from build123d import *

# Parameters (mm, degrees)
F2_DEPTH = 70


# Not quite as in the source:
# - ends of sketch curves that miss each other by under 0.0002 mm in the source are joined


with BuildPart() as f2:
    # F1 (on Front) → F2 (new body, symmetric)
    with BuildSketch(Plane.XZ):
        with BuildLine():
            Line((8.249944, 9.6642), (4.58573, 5.999986))
            Line((4.58573, 5.999986), (0.653534, 5.999986))
            ThreePointArc((0.653534, 5.999986), (0.5241245494, 5.9829489324), (0.4035341291, 5.9329987764))
            Line((0.4035341291, 5.9329987764), (-5.6e-05, 5.699986))
            Line((-5.6e-05, 5.699986), (-0.403646, 5.932999))
            ThreePointArc((-0.403646, 5.932999), (-0.653646, 5.999986), (-0.9036458709, 5.9329987764))
            Line((-0.9036458709, 5.9329987764), (-1.218942, 5.750963))
            Line((-1.218942, 5.750963), (-2.500056, 5.999986))
            Line((-2.500056, 5.999986), (-4.585842, 5.999986))
            Line((-4.585842, 5.999986), (-8.250056, 9.6642))
            Line((-8.250056, 9.6642), (-8.250056, 12.999986))
            Line((-8.250056, 12.999986), (-4.300056, 12.999986))
            ThreePointArc((-4.300056, 12.999986), (-4.0879239656, 13.0878539656), (-4.000056, 13.299986))
            Line((-4.000056, 13.299986), (-4.000056, 14.699986))
            ThreePointArc((-4.000056, 14.699986), (-4.0879239656, 14.9121180344), (-4.300056, 14.999986))
            Line((-4.300056, 14.999986), (-13.000056, 14.999986))
            ThreePointArc((-13.000056, 14.999986), (-14.4142695624, 14.4141995624), (-15.000056, 12.999986))
            Line((-15.000056, 12.999986), (-15.000056, 4.299986))
            ThreePointArc((-15.000056, 4.299986), (-14.9121880344, 4.0878539656), (-14.700056, 3.999986))
            Line((-14.700056, 3.999986), (-13.300056, 3.999986))
            ThreePointArc((-13.300056, 3.999986), (-13.0879239656, 4.0878539656), (-13.000056, 4.299986))
            Line((-13.000056, 4.299986), (-13.000056, 8.249986))
            Line((-13.000056, 8.249986), (-9.66427, 8.249986))
            Line((-9.66427, 8.249986), (-6.000056, 4.585772))
            Line((-6.000056, 4.585772), (-6.000056, 0.653576))
            ThreePointArc((-6.000056, 0.653576), (-5.9830189324, 0.5241665494), (-5.9330687764, 0.4035761291))
            Line((-5.9330687764, 0.4035761291), (-5.700056, -1.4e-05))
            Line((-5.700056, -1.4e-05), (-5.933069, -0.403604))
            ThreePointArc((-5.933069, -0.403604), (-6.000056, -0.653604), (-5.9330687764, -0.9036038709))
            Line((-5.9330687764, -0.9036038709), (-5.751033, -1.2189))
            Line((-5.751033, -1.2189), (-6.000056, -2.500014))
            Line((-6.000056, -2.500014), (-6.000056, -4.5858))
            Line((-6.000056, -4.5858), (-9.66427, -8.250014))
            Line((-9.66427, -8.250014), (-13.000056, -8.250014))
            Line((-13.000056, -8.250014), (-13.000056, -4.300014))
            ThreePointArc((-13.000056, -4.300014), (-13.0879239656, -4.0878819656), (-13.300056, -4.000014))
            Line((-13.300056, -4.000014), (-14.700056, -4.000014))
            ThreePointArc((-14.700056, -4.000014), (-14.9121880344, -4.0878819656), (-15.000056, -4.300014))
            Line((-15.000056, -4.300014), (-15.000056, -13.000014))
            ThreePointArc((-15.000056, -13.000014), (-14.4142695624, -14.4142275624), (-13.000056, -15.000014))
            Line((-13.000056, -15.000014), (12.999944, -15.000014))
            ThreePointArc((12.999944, -15.000014), (14.4141575624, -14.4142275624), (14.999944, -13.000014))
            Line((14.999944, -13.000014), (14.999944, -4.300014))
            ThreePointArc((14.999944, -4.300014), (14.9120760344, -4.0878819656), (14.699944, -4.000014))
            Line((14.699944, -4.000014), (13.299944, -4.000014))
            ThreePointArc((13.299944, -4.000014), (13.0878119656, -4.0878819656), (12.999944, -4.300014))
            Line((12.999944, -4.300014), (12.999944, -8.250014))
            Line((12.999944, -8.250014), (9.664158, -8.250014))
            Line((9.664158, -8.250014), (5.999944, -4.5858))
            Line((5.999944, -4.5858), (5.999944, -0.653604))
            ThreePointArc((5.999944, -0.653604), (5.9829069324, -0.5241945494), (5.9329567764, -0.4036041291))
            Line((5.9329567764, -0.4036041291), (5.699944, -1.4e-05))
            Line((5.699944, -1.4e-05), (5.932957, 0.403576))
            ThreePointArc((5.932957, 0.403576), (5.999944, 0.653576), (5.9329567764, 0.9035758709))
            Line((5.9329567764, 0.9035758709), (5.750921, 1.218872))
            Line((5.750921, 1.218872), (5.999944, 2.499986))
            Line((5.999944, 2.499986), (5.999944, 4.585772))
            Line((5.999944, 4.585772), (9.664158, 8.249986))
            Line((9.664158, 8.249986), (12.999944, 8.249986))
            Line((12.999944, 8.249986), (12.999944, 4.299986))
            ThreePointArc((12.999944, 4.299986), (13.0878119656, 4.0878539656), (13.299944, 3.999986))
            Line((13.299944, 3.999986), (14.699944, 3.999986))
            ThreePointArc((14.699944, 3.999986), (14.9120760344, 4.0878539656), (14.999944, 4.299986))
            Line((14.999944, 4.299986), (14.999944, 12.999986))
            ThreePointArc((14.999944, 12.999986), (14.4141575624, 14.4141995624), (12.999944, 14.999986))
            Line((12.999944, 14.999986), (4.299944, 14.999986))
            ThreePointArc((4.299944, 14.999986), (4.0878119656, 14.9121180344), (3.999944, 14.699986))
            Line((3.999944, 14.699986), (3.999944, 13.299986))
            ThreePointArc((3.999944, 13.299986), (4.0878119656, 13.0878539656), (4.299944, 12.999986))
            Line((4.299944, 12.999986), (8.249944, 12.999986))
            Line((8.249944, 12.999986), (8.249944, 9.6642))
        make_face()
        with BuildLine():
            Line((-4.171629, -6.000014), (4.171517, -6.000014))
            ThreePointArc((4.171517, -6.000014), (4.5542004324, -6.0761344675), (4.8786237812, -6.2929072188))
            Line((4.8786237812, -6.2929072188), (7.742837, -9.157121))
            ThreePointArc((7.742837, -9.157121), (8.0672605676, -9.3738935325), (8.449944, -9.450014))
            Line((8.449944, -9.450014), (11.073348, -9.450014))
            Line((11.073348, -9.450014), (12.349782, -9.914598))
            ThreePointArc((12.349782, -9.914598), (13.2040603505, -12.8608903949), (10.1374570291, -12.7810479799))
            ThreePointArc((10.1374570291, -12.7810479799), (9.3136995047, -12.3500149751), (8.4911490608, -12.7833470418))
            ThreePointArc((8.4911490608, -12.7833470418), (8.3119125635, -12.9425444809), (8.079175, -13.000014))
            Line((8.079175, -13.000014), (-8.079287, -13.000014))
            ThreePointArc((-8.079287, -13.000014), (-8.3120245635, -12.9425444809), (-8.4912608636, -12.7833469062))
            ThreePointArc((-8.4912608636, -12.7833469062), (-9.3138115047, -12.3500149751), (-10.1375690315, -12.7810479782))
            ThreePointArc((-10.1375690315, -12.7810479782), (-13.2041723505, -12.8608903949), (-12.3498940253, -9.9145979306))
            Line((-12.3498940253, -9.9145979306), (-11.07346, -9.450014))
            Line((-11.07346, -9.450014), (-8.450056, -9.450014))
            ThreePointArc((-8.450056, -9.450014), (-8.0673725676, -9.3738935325), (-7.7429492188, -9.1571207812))
            Line((-7.7429492188, -9.1571207812), (-4.878736, -6.292907))
            ThreePointArc((-4.878736, -6.292907), (-4.5543124324, -6.0761344675), (-4.171629, -6.000014))
        make_face(mode=Mode.SUBTRACT)
        with BuildLine():
            ThreePointArc((-12.3498940253, 9.9145699306), (-13.0435588843, 13.0434888843), (-9.9146399306, 12.3498240253))
            Line((-9.9146399306, 12.3498240253), (-9.547908, 11.342236))
            ThreePointArc((-9.547908, 11.342236), (-9.8735275063, 9.8734575063), (-11.3423061215, 9.5478376661))
            Line((-11.3423061215, 9.5478376661), (-12.3498940253, 9.9145699306))
        make_face(mode=Mode.SUBTRACT)
        with BuildLine():
            ThreePointArc((0.9882629956, -3.2532009855), (-5.6e-05, -3.400014), (-0.9883749956, -3.2532009855))
            ThreePointArc((-0.9883749956, -3.2532009855), (-1.3178396431, -3.2974811593), (-1.5000564258, -3.5755229349))
            ThreePointArc((-1.5000564258, -3.5755229349), (-1.6685571025, -3.8793255231), (-1.994322, -4.000014))
            Line((-1.994322, -4.000014), (-3.500056, -4.000014))
            ThreePointArc((-3.500056, -4.000014), (-3.8536093906, -3.8535673906), (-4.000056, -3.500014))
            Line((-4.000056, -3.500014), (-4.000056, -1.99428))
            ThreePointArc((-4.000056, -1.99428), (-3.8793675231, -1.6685151025), (-3.5755649263, -1.5000144822))
            ThreePointArc((-3.5755649263, -1.5000144822), (-3.2975231593, -1.3177976431), (-3.2532441585, -0.9883290481))
            ThreePointArc((-3.2532441585, -0.9883290481), (-3.400056, -1.4e-05), (-3.2532429855, 0.9883049956))
            ThreePointArc((-3.2532429855, 0.9883049956), (-3.2975231593, 1.3177696431), (-3.5755649349, 1.4999864258))
            ThreePointArc((-3.5755649349, 1.4999864258), (-3.8793675231, 1.6684871025), (-4.000056, 1.994252))
            Line((-4.000056, 1.994252), (-4.000056, 3.499986))
            ThreePointArc((-4.000056, 3.499986), (-3.8536093906, 3.8535393906), (-3.500056, 3.999986))
            Line((-3.500056, 3.999986), (-1.994322, 3.999986))
            ThreePointArc((-1.994322, 3.999986), (-1.6685571025, 3.8792975231), (-1.5000564822, 3.5754949263))
            ThreePointArc((-1.5000564822, 3.5754949263), (-1.3178396431, 3.2974531593), (-0.9883710481, 3.2531741585))
            ThreePointArc((-0.9883710481, 3.2531741585), (-5.6e-05, 3.399986), (0.9882629956, 3.2531729855))
            ThreePointArc((0.9882629956, 3.2531729855), (1.3177276431, 3.2974531593), (1.4999444258, 3.5754949349))
            ThreePointArc((1.4999444258, 3.5754949349), (1.6684451025, 3.8792975231), (1.99421, 3.999986))
            Line((1.99421, 3.999986), (3.499944, 3.999986))
            ThreePointArc((3.499944, 3.999986), (3.8534973906, 3.8535393906), (3.999944, 3.499986))
            Line((3.999944, 3.499986), (3.999944, 1.994252))
            ThreePointArc((3.999944, 1.994252), (3.8792555231, 1.6684871025), (3.5754529263, 1.4999864822))
            ThreePointArc((3.5754529263, 1.4999864822), (3.2974111593, 1.3177696431), (3.2531321585, 0.9883010481))
            ThreePointArc((3.2531321585, 0.9883010481), (3.399944, -1.4e-05), (3.2531309855, -0.9883329956))
            ThreePointArc((3.2531309855, -0.9883329956), (3.2974111593, -1.3177976431), (3.5754529349, -1.5000144258))
            ThreePointArc((3.5754529349, -1.5000144258), (3.8792555231, -1.6685151025), (3.999944, -1.99428))
            Line((3.999944, -1.99428), (3.999944, -3.500014))
            ThreePointArc((3.999944, -3.500014), (3.8534973906, -3.8535673906), (3.499944, -4.000014))
            Line((3.499944, -4.000014), (1.99421, -4.000014))
            ThreePointArc((1.99421, -4.000014), (1.6684451025, -3.8793255231), (1.4999444822, -3.5755229263))
            ThreePointArc((1.4999444822, -3.5755229263), (1.3177276431, -3.2974811593), (0.9882629956, -3.2532009855))
        make_face(mode=Mode.SUBTRACT)
        with BuildLine():
            ThreePointArc((11.3421941215, 9.5478376661), (9.8734155063, 9.8734575063), (9.5477956661, 11.3422361215))
            Line((9.5477956661, 11.3422361215), (9.914528, 12.349824))
            ThreePointArc((9.914528, 12.349824), (13.0434468843, 13.0434888843), (12.3497820253, 9.9145699306))
            Line((12.3497820253, 9.9145699306), (11.3421941215, 9.5478376661))
        make_face(mode=Mode.SUBTRACT)
    extrude(amount=F2_DEPTH, both=True)


solid = f2.part
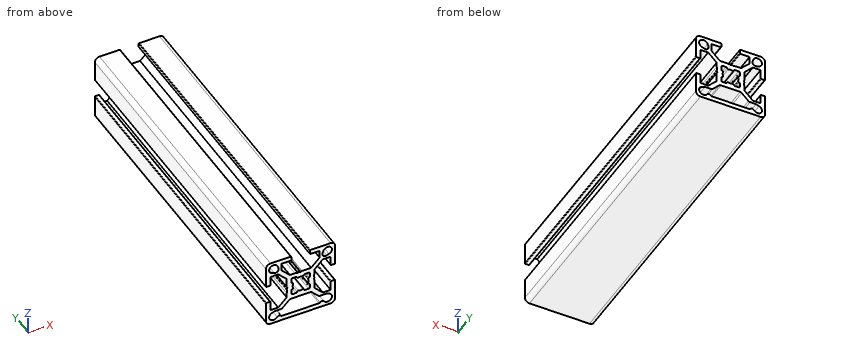
Source: CAD feature listing. Evaluate the final solid. Frame: model axes, mm. Round coordinates to 2 decimals unless told otherwise and drop trailing zeros. One line per item, written item: value. Start each with the question number.
Item 1: Pin query (flat end, axial travel): pin 1 (5 mm diameter, centred on y = 40.5, z = 0.5, fed in from +X); pin 2 (1.7 mm diameter, centred on y = 17.5, z = -2.5, fed in from -X); pin 3 (1.1 mm diameter, centred on y = 20, z = 14, fed in from +X); pin 4 (1 mm diameter, centred on x = -7.5, z = -2.5, fed in from +Y). Return the tip coordinate at first contact, or that it passes through.
Item 2: Section query A-A (y = -23). State how many separate pieces and enclosed holes the cut face has, plus the area to 3 significant figures.
Item 3: Ray query, L1, parallel to Z at x = -3, y = -59; L2, parallel to X at y = 10.5, z = -12.75; L3, parallel to Z at x = 10.5, y = 15. Return the intervals inside material, ascending. Write a range as from..to.
Result set:
1. pin 1: stops at x = 6
1. pin 2: stops at x = -6
1. pin 3: stops at x = 14.95
1. pin 4: passes through
2. separate pieces: 1
2. enclosed holes: 4
2. area: 322 mm²
3. L1: z = -15..-13, -6..-4, 4..6
3. L2: x = -15..-13.28, -10.12..-8.52, 8.52..10.12, 13.28..15
3. L3: z = -15..-13.17, -9.45..-8.25, 8.25..9.51, 13.17..15
